Answer from the drawing. Dimensions are ordinates in mm from the lowest x, y and z of the part. A direction names the side the tool comes from. Coordinates: 2 decimals unless noted, no trailing zeros. Write each loop counter-clockwise with the first axis right and the second up, starting at its lowest first coordinate (ties: lowest second). Pieces come first, ordered by that corner, then holes.
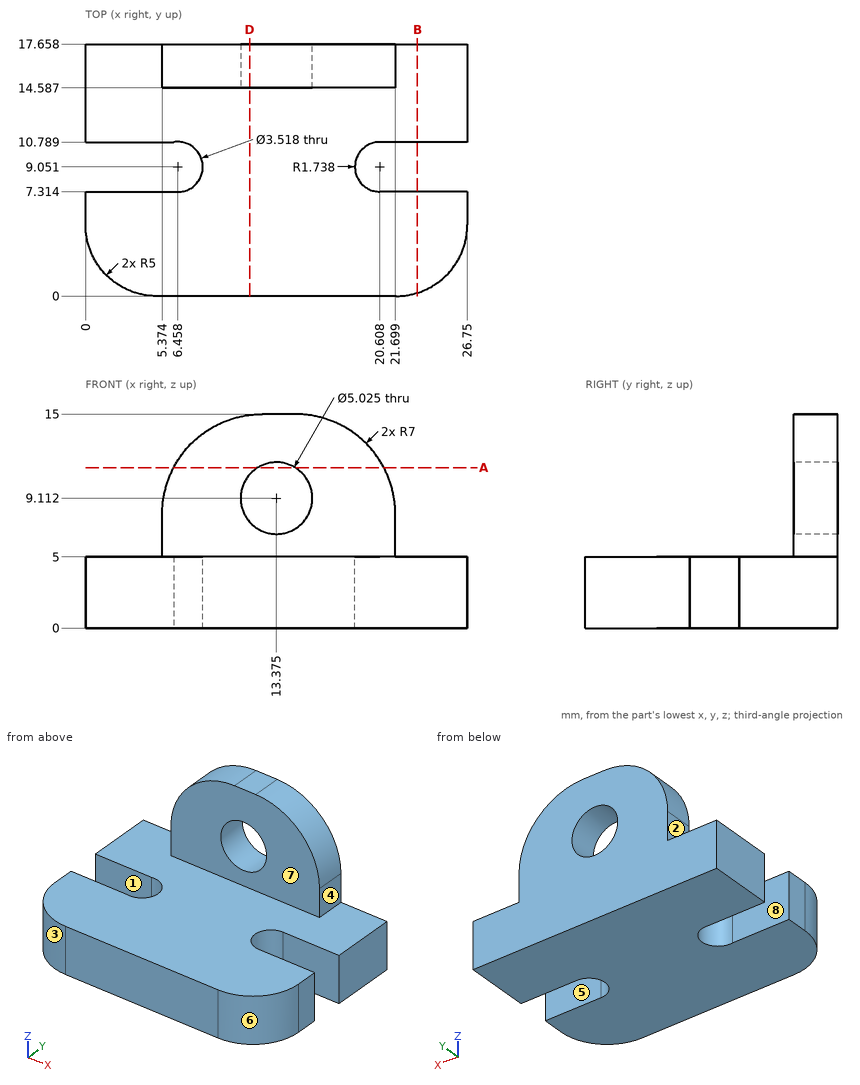
(1) Which of the six approach directions +Z, -Z, +X, -X, +Y, -Y give full straight-line access (tool end or side, diameter ignored) to the marked faces 4, 5, 6, 7 and 8?
(2) For a pull along Y with two mould halves and no side action, classify the marked faces 1, 2 and 3 as pulls with the +Y half, pulls with the -Y half, needs draft (parallel to the pull), parting line crosses it, or undercut.
(3) Section D-D, the plane x = 11.5 is taken. Write down the section's boundary in (y, z) (1 decimal), plus the area to 3 significant figures.
(4) Section B-B, the plane x = 23.25 is taken. Write down the section's boundary in (y, z).
(5) Section A-A, the plane z = 11.25 is taken. Write down the section's boundary in (x, y) (1 decimal).
(6) Each of these flat-tipped pins is pushed along its axis until it touches: pin 1 (5.5 mm diameter, centred on x = 17.5, y = 4.5, fed in from +Z); pin 2 (2.5 mm diameter, centred on x = 25, z = 3.5, fed in from -Y); pin 3 (2.5 mm diameter, centred on x = 2.5, z = 3, fed in from -Y); pin 4 (2 mm diameter, centred on x = 6.46, y = 9.05, fed in from -Z). Where does it stop, or does it pass through?
(7) Find the intervals of material crossed by probe 1 along Y at (x, z) = (5.75, 2); probe 2 along Z at (x, y) = (23.5, 5.75); probe 3 along Y at (x, z) = (9.25, 6.75), in increasing order.
Solution:
1. face 4: +Z, +X, +Y, -Y
1. face 5: +Z, -Z, +X
1. face 6: +Z, -Z, +X, -Y
1. face 7: +Z, +X, -X, -Y
1. face 8: +Z, -Z, -X
2. face 1: undercut
2. face 2: needs draft
2. face 3: pulls with the -Y half
3. outline: (0, 0) - (17.7, 0) - (17.7, 7.4) - (14.6, 7.4) - (14.6, 5) - (0, 5) - close; (14.6, 10.8) - (17.7, 10.8) - (17.7, 14.9) - (14.6, 14.9) - close
3. area: 109 mm2
4. outline: (0.23, 0) - (7.31, 0) - (7.31, 5) - (0.23, 5) - close; (10.79, 0) - (17.66, 0) - (17.66, 5) - (10.79, 5) - close
5. outline: (6.2, 14.6) - (12.1, 14.6) - (12.1, 17.7) - (6.2, 17.7) - close; (14.7, 14.6) - (20.9, 14.6) - (20.9, 17.7) - (14.7, 17.7) - close
6. pin 1: stops at z = 5
6. pin 2: stops at y = 0.42
6. pin 3: stops at y = 0.16
6. pin 4: passes through
7. probe 1: y = 0 to 7.31, 10.79 to 17.66
7. probe 2: z = 0 to 5
7. probe 3: y = 14.59 to 17.66
